```python
from build123d import *

# Parameters (mm, degrees)
AUFSATZ_LINEAR_AUSTRAGEN1_DEPTH                      = 6
SKIZZE1_4_R                                          = 25
SCHNITT_LINEAR_AUSTRAGEN1_DEPTH                      = 2
SKIZZE1_5_R                                          = 17
SCHNITT_LINEAR_AUSTRAGEN2_DEPTH                      = 142.529148941
SKIZZE1_6_R                                          = 2.25
SCHNITT_LINEAR_AUSTRAGEN3_DEPTH                      = 142.529148941
CSK_FOR_M3_RAISED_COUNTERSUNK_HEAD_SCREW_D           = 3.4
CSK_FOR_M3_RAISED_COUNTERSUNK_HEAD_SCREW_DEPTH       = 10
CSK_FOR_M3_RAISED_COUNTERSUNK_HEAD_SCREW_CSINK_D     = 4
CSK_FOR_M3_RAISED_COUNTERSUNK_HEAD_SCREW_CSINK_ANGLE = 90
CSK_FOR_M3_RAISED_COUNTERSUNK_HEAD_SCREW_TIP         = 1.021463052


with BuildPart() as part:
    # Skizze1 → Aufsatz-Linear austragen1 (new body)
    with BuildSketch(Plane(origin=(0, 0, 0), x_dir=(1, 0, 0), z_dir=(0, 1, 0))):
        with BuildLine():
            Line((0, 0), (-28.5, 0))
            Line((-28.5, 0), (-28.5, 110))
            ThreePointArc((-28.5, 110), (0, 138.5), (28.5, 110))
            Line((28.5, 110), (28.5, 0))
            Line((28.5, 0), (0, 0))
        make_face()
    extrude(amount=AUFSATZ_LINEAR_AUSTRAGEN1_DEPTH)

    # Skizze1_4 → Schnitt-Linear austragen1 (cut)
    with BuildSketch(Plane(origin=(0, 0, 0), x_dir=(1, 0, 0), z_dir=(0, 1, 0))):
        with Locations(Location((0, 110, 0), (0, 0, 270))):
            Circle(SKIZZE1_4_R)
    extrude(amount=SCHNITT_LINEAR_AUSTRAGEN1_DEPTH, mode=Mode.SUBTRACT)

    # Skizze1_5 → Schnitt-Linear austragen2 (cut, through all)
    with BuildSketch(Plane(origin=(0, 0, 0), x_dir=(1, 0, 0), z_dir=(0, 1, 0))):
        with Locations(Location((0, 110, 0), (0, 0, 270))):
            Circle(SKIZZE1_5_R)
    extrude(amount=SCHNITT_LINEAR_AUSTRAGEN2_DEPTH, mode=Mode.SUBTRACT)

    # Skizze1_6 → Schnitt-Linear austragen3 (cut, through all)
    with BuildSketch(Plane(origin=(0, 0, 0), x_dir=(1, 0, 0), z_dir=(0, 1, 0))):
        with Locations(Location((14.849242405, 95.150757595, 0), (0, 0, 270))):
            Circle(SKIZZE1_6_R)
        with Locations(Location((-20.284442352, 104.564800053, 0), (0, 0, 270))):
            Circle(SKIZZE1_6_R)
        with Locations(Location((5.435199947, 130.284442352, 0), (0, 0, 270))):
            Circle(SKIZZE1_6_R)
    extrude(amount=SCHNITT_LINEAR_AUSTRAGEN3_DEPTH, mode=Mode.SUBTRACT)

    # CSK for M3 Raised Countersunk Head Screw
    with Locations(Plane(origin=(-24, 3, 0), x_dir=(1, 0, 0), z_dir=(0, 0, 1))):
        with Locations((0, 0), (11, 0), (37, 0), (48, 0)):
            CounterSinkHole(CSK_FOR_M3_RAISED_COUNTERSUNK_HEAD_SCREW_D / 2, CSK_FOR_M3_RAISED_COUNTERSUNK_HEAD_SCREW_CSINK_D / 2, depth=CSK_FOR_M3_RAISED_COUNTERSUNK_HEAD_SCREW_DEPTH, counter_sink_angle=CSK_FOR_M3_RAISED_COUNTERSUNK_HEAD_SCREW_CSINK_ANGLE)
            with Locations((0, 0, -(CSK_FOR_M3_RAISED_COUNTERSUNK_HEAD_SCREW_DEPTH + CSK_FOR_M3_RAISED_COUNTERSUNK_HEAD_SCREW_TIP / 2))):  # 118° drill point
                Cone(0, CSK_FOR_M3_RAISED_COUNTERSUNK_HEAD_SCREW_D / 2, CSK_FOR_M3_RAISED_COUNTERSUNK_HEAD_SCREW_TIP, mode=Mode.SUBTRACT)


solid = part.part
```
The listing builds one solid part. Answer for the finished solid, in the listing's coordinates (mm). A direction names the side the tool comes from. Give positions to 0.01 mm unless a question says otherwise; leave off trailing zeros. Order: outer loops, then holes, each group sorted by start corner. A loop starts at its lowest first (then second) coordinate and runs counter-clockwise, first axis right, second up. Notation, with made-up numbers: (78.25, -11.5) - (98.25, -11.5) arc R18 cw to (98.25, 23.5) - close; hole circle Ø6 at (30.25, 41.5). An arc over 180 degrees is marked (long way). Answer in a Markdown table with one row per item. Add a question column.
Q1. The part is cut by section A-A (z = -119.5). Determine the outline of the cut face in (x, y), then the cut area to 3 significant figures.
Q2. Find the intervals of material crossed by line 1 along X through (y, z) = (3, -3); line 2 along Z through (x, y) = (0, 3.35); line 3 along Y through (x, z) = (-13, -7.25), in increasing order. Write a range as [from, to].
Q3. Given P1, Ø15, axis at x = 2, z = -104, coming from the -Y side; P2, Ø2, axis at x = -24, y = 3, coming from the +Z side; P3, Ø1.5, axis at x = -5, y = 2, coming from the +Z side; P4, Ø1, axis at y = 2, z = -118.5, coming from the +X side, each flat-ended and moving along its own axis, determine where each tip first touches the part or whether it passes through.
Q4. Which of the six approach directions +Z, -Z, +X, -X, +Y, -Y give full straight-line access (tool end or side, diameter ignored) to faces 4 (the flat face through (5.9, 2, -93.7)), 5 (the cylindrical face through (-21.15, 3.97, -102.49)), 6 (the cylindrical face through (11.38, 3.51, -5.22))?
Q5. For a pull along Y with two mould halves and no side action, classify faces 1 (the flat face through (0, 3, 0)), 2 (the flat face through (0, 6, -55)), 3 (the cylindrical face through (22.43, 2.35, -5.22)) as released by +Y, released by -Y, zero draft, split by the parting line, or undercut.
Determined:
| question | item | result |
|---|---|---|
| 1 | outline | (-26.87, 0) - (-23.12, 0) - (-23.12, 2) - (-14.1, 2) - (-14.1, 6) - (-26.87, 6) - close; (14.1, 2) - (23.12, 2) - (23.12, 0) - (26.87, 0) - (26.87, 6) - (14.1, 6) - close |
| 1 | area | 117 mm² |
| 2 | line 1 | x = [-28.5, -25.7], [-22.3, -14.7], [-11.3, 11.3], [14.7, 22.3], [25.7, 28.5] |
| 2 | line 2 | z = [-138.5, -127], [-93, 0] |
| 2 | line 3 | y = [0, 1.3], [4.7, 6] |
| 3 | P1 | passes through |
| 3 | P2 | stops at z = -10.42 |
| 3 | P3 | stops at z = 0 |
| 3 | P4 | stops at x = 27.35 |
| 4 | face 4 | -Y |
| 4 | face 5 | +Y, -Y |
| 4 | face 6 | +Z |
| 5 | face 1 | zero draft |
| 5 | face 2 | released by +Y |
| 5 | face 3 | undercut |
